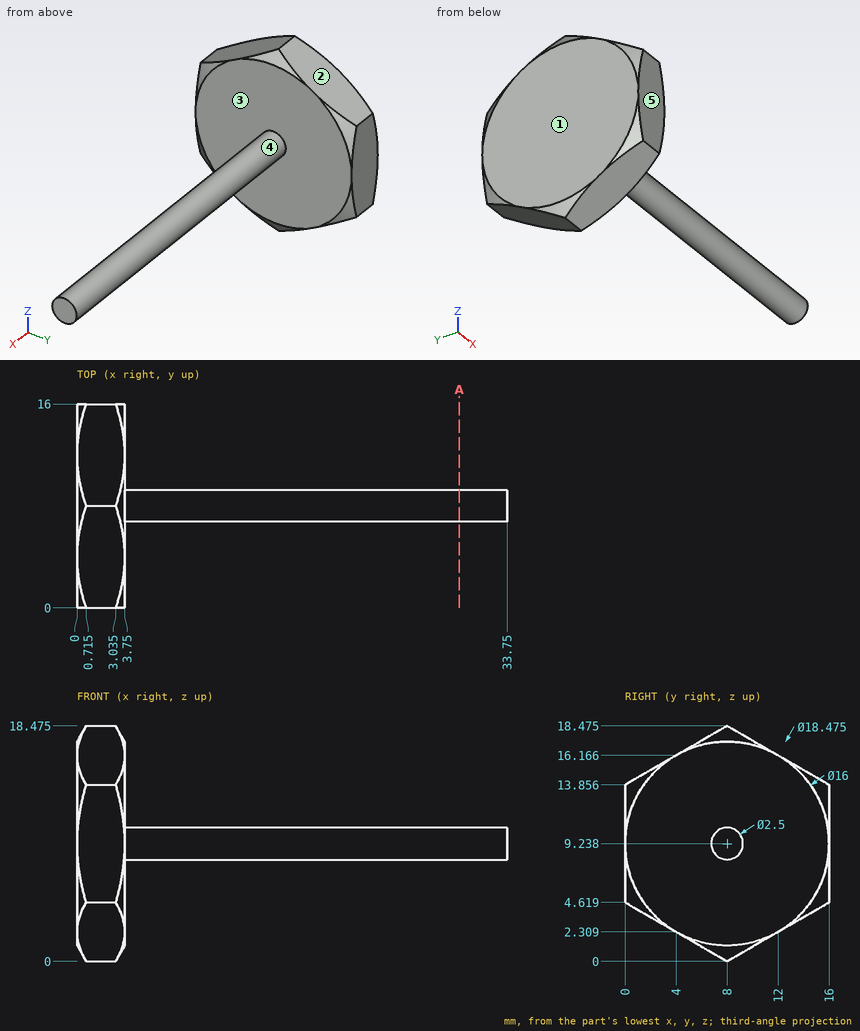
Print and shaded views of the part. All mm, measured from the part's lowest x, y and z. A direction names the side the tool comes from. Coordinates: 2 decimals unless noted, no trailing zeros. Order: outer loops, then holes, each group sorted by start corner. A loop starts at its lowest first (then second) coordinate and runs counter-clockwise, first axis right, second up.
Item 1: Drop flat-ended pins along their axis: pin 1 Ø5 at (x, y) = (9.5, 5.5) entering from -Z; pin 2 Ø1.5 at (x, z) = (3.5, 15) entering from -Y (1 decimal). Give the stop position or say it passes through.
Filled in:
pin 1: stops at z = 7.99
pin 2: stops at y = 0.7
Item 2: Saw through at A-A on x = 30. List the corners of the cut face in (y, z).
Filled in:
outline: circle Ø2.5 at (8, 9.24)
Item 3: Drill centre lines: L1, parallel to X at y = 11.25, z = 5.75; L2, parallel to Y at x = 28, z = 9.25; L3, parallel to Z at x = 25, y = 9 (1 decimal). Where is each one in solid material? Low to high.
Filled in:
L1: x = 0 to 3.75
L2: y = 6.75 to 9.25
L3: z = 8.5 to 10
Item 4: Mould opens along X. For the marked faces 1, 2 and 3 say: released by +X, released by -X, zero draft, split by the parting line, or undercut.
Filled in:
face 1: released by -X
face 2: zero draft
face 3: released by +X
Item 5: Tool access for the marked faces 4 and 5: list every direction of +Z, -Z, +X, -X, +Y, -Y with a clear straight run to the whole face (end or side of a thin tool).
Filled in:
face 4: +X
face 5: +Z, -Z, +X, -X, -Y
